Design review of the part built by this model. Coordinates are the model's own, in mm. A direction names the side the tool comes from. Coordinates: 2 decimals unless noted, no trailing zeros. Write each loop counter-clockwise with the first axis right and the second up, starting at its lowest first coordinate (ties: lowest second). Pieces come first, ordered by that corner, then holes. Notation, with made-up numbers: (57.5, 36.5) -> (72.5, 36.5) arc R5 cw to (72.5, 45.5) -> close; hole circle Ø8 at (-39.75, -29). An arc over 180 degrees is marked (long way). Answer in a Markdown table with one row per item. Add a question column.
Item 1: Take a section at C-C, the plane x = -5. Write out the cut boundary in (y, z), and give its area (3 significant figures).
Item 2: Take a section at A-A, the plane z = -4.5. Write out the cut boundary in (x, y).
Item 3: For faces 1 (the face through (39, 18, 52.51)), 2 (the face through (-31, 7, 42.51)), 3 (the face through (4, 0, -39)), 4 (the face through (39, 15, -7)), list the 3-axis set-ups (+Z, -Z, +X, -X, +Y, -Y) from which the entire face can be reached by the end or side of a thin tool; tool diameter is ignored.
Item 4: To check wall thickness, follow line 1 (X direction, y = 31, z = 4.5); line 2 (Y direction, x = -17, z = -45); line 3 (Z direction, x = -15.5, y = 8.5). State the ranges of each line that lie inside material, in increasing order.
Item 5: Clearance check with flat-ended pins moving along their axes: P1, Ø10, axis at x = -8, y = 16.5, coming from the -Z side; P2, Ø8, axis at x = -0.5, z = 48.5, coming from the +Y side; P3, Ø1.5, axis at x = -30, y = 29.5, coming from the +Z side; P4, Ø4, axis at x = -22, y = 1.5, coming from the +Z side. State where each tip first meets the part, or that it passes through.
Item 6: Take a section at B-B, the plane y = 2. Write out the cut boundary in (x, z).
Item 7: Take a section at D-D, the plane x = -23. Write out the cut boundary in (y, z).
Item 8: Draft analysis for pull direction X (two halves, no side actions). For faces 5 (the face through (4, -2.5, 38)), 6 (the face through (6, 18, -17.49)), 7 (the face through (-33.178, 17, 19)), state which applies: released by +X, released by -X, zero draft, split by the parting line, or undercut.
from build123d import *

# Parameters (mm, degrees)
SKETCH3_W           = 75
SKETCH3_H           = 85
BOSS_EXTRUDE1_DEPTH = 35
SKETCH4_W           = 65
SKETCH4_H           = 75
CUT_EXTRUDE1_DEPTH  = 40
SKETCH8_W           = 75
SKETCH8_H           = 150
BOSS_EXTRUDE2_DEPTH = 2.5
SKETCH9_R           = 15
CUT_EXTRUDE4_DEPTH  = 15
SKETCH10_W          = 75
SKETCH10_H          = 33.016749553
CUT_EXTRUDE5_DEPTH  = 10
SKETCH16_W          = 20
SKETCH16_H          = 15
CUT_EXTRUDE6_DEPTH  = 10
SKETCH17_W          = 10
SKETCH17_H          = 1.983250447
CUT_EXTRUDE7_DEPTH  = 66
SKETCH19_W          = 20
SKETCH19_H          = 15
CUT_EXTRUDE8_DEPTH  = 10


with BuildPart() as part:
    # Sketch3 → Boss-Extrude1 (new body)
    with BuildSketch(Plane(origin=(0, 0, 0), x_dir=(1, 0, 0), z_dir=(0, 1, 0))):
        with Locations((4.321862348, -20.010121457)):
            Rectangle(SKETCH3_W, SKETCH3_H)
    extrude(amount=BOSS_EXTRUDE1_DEPTH)

    # Sketch4 → Cut-Extrude1 (cut)
    with BuildSketch(Plane(origin=(0, 35, 0), x_dir=(1, 0, 0), z_dir=(0, 1, 0))):
        with Locations((4.321862348, -20.010121457)):
            Rectangle(SKETCH4_W, SKETCH4_H)
    extrude(amount=-CUT_EXTRUDE1_DEPTH, mode=Mode.SUBTRACT)

    # Sketch8 → Boss-Extrude2 (add)
    with BuildSketch(Plane.XZ):
        with Locations((4.321862348, 20.010121457)):
            Rectangle(SKETCH8_W, SKETCH8_H)
    extrude(amount=BOSS_EXTRUDE2_DEPTH)

    # Sketch9 → Cut-Extrude4 (cut)
    with BuildSketch(Plane.XZ.offset(2.5)):
        with Locations((4.321862348, 20.010121457)):
            Circle(SKETCH9_R)
    extrude(amount=-CUT_EXTRUDE4_DEPTH, mode=Mode.SUBTRACT)

    # Sketch10 → Cut-Extrude5 (cut)
    with BuildSketch(Plane.XY.offset(62.510121457)):
        with Locations((4.321862348, 18.491625224)):
            Rectangle(SKETCH10_W, SKETCH10_H)
    extrude(amount=-CUT_EXTRUDE5_DEPTH, mode=Mode.SUBTRACT)

    # Sketch16 → Cut-Extrude6 (cut)
    with BuildSketch(Plane.ZY.offset(33.178137652)):
        with Locations((52.510121457, 7.5)):
            Rectangle(SKETCH16_W, SKETCH16_H)
    extrude(amount=-CUT_EXTRUDE6_DEPTH, mode=Mode.SUBTRACT)

    # Sketch17 → Cut-Extrude7 (cut, through all)
    with BuildSketch(Plane.ZY.offset(23.178137652)):
        with Locations((57.510121457, 0.991625224)):
            Rectangle(SKETCH17_W, SKETCH17_H)
    extrude(amount=-CUT_EXTRUDE7_DEPTH, mode=Mode.SUBTRACT)

    # Sketch19 → Cut-Extrude8 (cut)
    with BuildSketch(Plane(origin=(41.821862348, 0, 0), x_dir=(0, 0, -1), z_dir=(1, 0, 0))):
        with Locations((7.489878543, 7.5)):
            Rectangle(SKETCH19_W, SKETCH19_H)
    extrude(amount=-CUT_EXTRUDE8_DEPTH, mode=Mode.SUBTRACT)


solid = part.part
Answers:
| question | item | result |
|---|---|---|
| 1 | outline | (-2.5, -54.99) -> (0, -54.99) -> (0, -22.49) -> (35, -22.49) -> (35, -17.49) -> (0, -17.49) -> (0, 8.26) -> (-2.5, 8.26) -> close; (-2.5, 31.76) -> (0, 31.76) -> (0, 95.01) -> (-2.5, 95.01) -> close |
| 1 | area | 491 mm^2 |
| 2 | outline | (-33.18, -2.5) -> (41.82, -2.5) -> (41.82, 0) -> (-28.18, 0) -> (-28.18, 35) -> (-33.18, 35) -> close; (36.82, 15) -> (41.82, 15) -> (41.82, 35) -> (36.82, 35) -> close |
| 3 | face 1 | +Z, +X, -X, +Y |
| 3 | face 2 | +Z, -X |
| 3 | face 3 | -Z, +X, -X, +Y |
| 3 | face 4 | +X |
| 4 | line 1 | x = -33.18 to -28.18, 36.82 to 41.82 |
| 4 | line 2 | y = -2.5 to 0 |
| 4 | line 3 | z = -22.49 to -17.49 |
| 5 | P1 | stops at z = -22.49 |
| 5 | P2 | stops at y = 0 |
| 5 | P3 | stops at z = 52.51 |
| 5 | P4 | stops at z = 95.01 |
| 6 | outline | (-33.18, -22.49) -> (41.82, -22.49) -> (41.82, -17.49) -> (-28.18, -17.49) -> (-28.18, 42.51) -> (-33.18, 42.51) -> close; (36.82, 2.51) -> (41.82, 2.51) -> (41.82, 52.51) -> (36.82, 52.51) -> close |
| 7 | outline | (-2.5, -54.99) -> (0, -54.99) -> (0, -22.49) -> (35, -22.49) -> (35, -17.49) -> (0, -17.49) -> (0, 95.01) -> (-2.5, 95.01) -> close |
| 8 | face 5 | zero draft |
| 8 | face 6 | undercut |
| 8 | face 7 | released by -X |
